Check sheet for the modelled part. Datum: model origin and axes. Units: mm. Give positions to 0.01 mm unless a question says otherwise; leave off trailing zeros. Loops run counter-clockwise (first coordinate to the right, second up) from the corner with the lowest first, then second, coordinate; pieces in that order, holes last. Notation, with made-up numbers: (-3.5, 5) - (4.5, 5) arc R34 cw to (4.5, 37) - close; hole circle Ø7 at (69, 3). An arc over 180 degrees is marked (long way). Use CSV: the item, a comma, the result in double quotes.
Autodesk Inventor part; units mm, degrees
ref_plane "YZ Plane" through (0, 0, 0) normal (1, 0, 0) x (0, 1, 0)
ref_plane "XZ Plane" through (0, 0, 0) normal (0, 1, 0) x (-1, 0, 0)
ref_plane "XY Plane" through (0, 0, 0) normal (0, 0, 1) x (1, 0, 0)
sketch "Base" plane through (0, 0, 0) normal (0, 0, 1) x (1, 0, 0)
  circle A0 centre (0, 0) radius 3.9873
  circle A1 centre (0, 0) radius 8.7406
  line L0 (-4.5, -4.5) -> (4.5, -4.5) construction
  line L1 (4.5, -4.5) -> (4.5, 4.5) construction
  line L2 (4.5, 4.5) -> (-4.5, 4.5) construction
  line L3 (-4.5, 4.5) -> (-4.5, -4.5) construction
  line L4 (-4.5, -4.5) -> (4.5, 4.5) construction
  line L5 (4.5, -4.5) -> (-4.5, 4.5) construction
  line L6 (-12.2369, 0) -> (12.2369, 0) construction
  circle A2 centre (0, 0) radius 6.364 construction
  circle A3 centre (-4.5, 4.5) radius 1.225
  circle A4 centre (4.5, 4.5) radius 1.225
  circle A5 centre (4.5, -4.5) radius 1.225
  circle A6 centre (-4.5, -4.5) radius 1.225
  dimension "d0" = 7.9746
  dimension "d1" = 4.7533
  dimension "d2" = 2.3767
  dimension "d3" = 2.45
  dimension "d4" = 9
extrude "Plate1" add sketch "Base" along normal blind 2
equation "\"d2\" = 0.5 * d1"
equation "\"d7\" = Thickness"
equation "\"BendRadius\" = Thickness"
equation "\"BendReliefWidth\" = Thickness"
equation "\"BendReliefDepth\" = 0.5 * Thickness"
equation "\"CornerReliefSize\" = 4 * Thickness"
equation "\"MinimumRemnant\" = 2 * Thickness"
equation "\"TransitionRadius\" = BendRadius"
equation "\"JacobiRadiusSize\" = BendRadius"
equation "\"GapSize\" = Thickness"
properties part number "WheelEncoderMagnetAlignmentFlange"
1. Sectioned sample at D-D, the plane x = 4.5. Record the boundary of the cut face in (y, z) (3 decimals).
Completed:
outline,"(-7.493, 0) - (-5.725, 0) - (-5.725, 2) - (-7.493, 2) - close; (-3.275, 0) - (3.275, 0) - (3.275, 2) - (-3.275, 2) - close; (5.725, 0) - (7.493, 0) - (7.493, 2) - (5.725, 2) - close"
2. Scan lines: line 1 along X through (y, z) = (-4.75, 1.55); line 2 along Y through (x, z) = (0, 1.5); line 3 along Y through (x, z) = (4.5, 0.5) (3 decimals). Record each from-to range of solid material in increasing order.
Completed:
line 1,"x = -7.34 to -5.7, -3.3 to 3.3, 5.7 to 7.34"
line 2,"y = -8.74 to -3.99, 3.99 to 8.74"
line 3,"y = -7.493 to -5.725, -3.275 to 3.275, 5.725 to 7.493"
3. Sectioned sample at A-A, the plane y = 0. Record the boundary of the cut face in (x, z).
Completed:
outline,"(-8.74, 0) - (-3.99, 0) - (-3.99, 2) - (-8.74, 2) - close; (3.99, 0) - (8.74, 0) - (8.74, 2) - (3.99, 2) - close"
4. Go/stop test with a flat-tipped pin: pin 1 Ø2 at (x, y) = (4.5, 4.5) entering from +Z. Record where the tip stops, or that it passes through.
Completed:
pin 1,"passes through"
5. Sectioned sample at C-C, the plane z = 1.45. Record the boundary of the cut face in (x, y) (3 decimals).
Completed:
outline,"circle Ø17.481 at (0, 0); hole circle Ø2.45 at (-4.5, -4.5); hole circle Ø2.45 at (-4.5, 4.5); hole circle Ø7.975 at (0, 0); hole circle Ø2.45 at (4.5, -4.5); hole circle Ø2.45 at (4.5, 4.5)"
6. Release check for a two-part mould opening along X. For faces 1 (the face through (-1.138, -8.666, 0.986)), 2 (the face through (4.234, 5.696, 0.986)), 3 (the face through (4, -2, 2)) record: released by +X, released by -X, zero draft, split by the parting line, or undercut.
Completed:
face 1,"split by the parting line"
face 2,"undercut"
face 3,"zero draft"
7. Sectioned sample at B-B, the plane x = -2.5. Record the boundary of the cut face in (y, z), and give its area (3 significant figures).
Completed:
outline,"(-8.38, 0) - (-3.11, 0) - (-3.11, 2) - (-8.38, 2) - close; (3.11, 0) - (8.38, 0) - (8.38, 2) - (3.11, 2) - close"
area,"21.1 mm²"
